```python
from build123d import *

# Parameters (mm, degrees)
SKETCH1_W                    = 44
SKETCH1_H                    = 210
BASE_FLANGE1_DEPTH           = 0.5
SKETCH6_R                    = 5
CUT_EXTRUDE1_DEPTH           = 108.281172626
LPATTERN1_COUNT              = 8
LPATTERN1_PITCH              = 25
EDGE_FLANGE1_STRIP_W         = 2.1
EDGE_FLANGE1_STRIP_H         = 0.5
EDGE_FLANGE1_STRIP_CUT_DEPTH = 210
EDGE_FLANGE1_DEPTH           = 210
F_7_0_7_DIAMETER_HOLE1_D     = 7
F_7_0_7_DIAMETER_HOLE1_DEPTH = 60
F_7_0_7_DIAMETER_HOLE1_TIP   = 2.103012167
BREAK_CORNER1_START          = 22
BREAK_CORNER1_DEPTH          = 0.5
CUT_EXTRUDE2_DEPTH           = 110.139818581
CUT_EXTRUDE2_DEPTH_BACK      = 110.139818581
SKETCH13_R                   = 3.1


# Read off the part's stored shape, not the designer's step: Break-Corner1
# Sheet-metal steps are written as plain solids
with BuildPart() as part:
    # Sketch1 → Base-Flange1 (new body)
    with BuildSketch(Plane.XY):
        Rectangle(SKETCH1_W, SKETCH1_H)
    extrude(amount=-BASE_FLANGE1_DEPTH)

    # Sketch6 → Cut-Extrude1 (cut, symmetric)
    with BuildSketch(Plane.XY):
        with Locations((10.825317547, 95)):
            Circle(SKETCH6_R)
        with Locations((-10.825317547, 82.5)):
            Circle(SKETCH6_R)
    cut_extrude1 = extrude(amount=CUT_EXTRUDE1_DEPTH, both=True, mode=Mode.SUBTRACT)

    # LPattern1: Cut-Extrude1 ×8
    with Locations(*[(0, -i * LPATTERN1_PITCH, 0) for i in range(1, LPATTERN1_COUNT)]):
        add(cut_extrude1, mode=Mode.SUBTRACT)

    # Edge-Flange1 strip (across the edge) → Edge-Flange1 strip cut (cut)
    with BuildSketch(Plane(origin=(22, -105, 0), x_dir=(-1, 0, 0), z_dir=(0, 1, 0))):
        with Locations((-1, -0.25)):
            Rectangle(EDGE_FLANGE1_STRIP_W, EDGE_FLANGE1_STRIP_H)
    extrude(amount=EDGE_FLANGE1_STRIP_CUT_DEPTH, mode=Mode.SUBTRACT)

    # Edge-Flange1 section (across the edge) → Edge-Flange1 (add)
    with BuildSketch(Plane(origin=(22, -105, 0), x_dir=(-1, 0, 0), z_dir=(0, 1, 0))):
        with BuildLine():
            Line((-0.5, 0.05), (-0.5, 19.5))
            Line((-0.5, 19.5), (0, 19.5))
            Line((0, 19.5), (0, 0.05))
            ThreePointArc((0, 0.05), (0.014644661, 0.014644661), (0.05, 0))
            Line((0.05, 0), (0.05, -0.5))
            ThreePointArc((0.05, -0.5), (-0.33890873, -0.33890873), (-0.5, 0.05))
        make_face()
    extrude(amount=EDGE_FLANGE1_DEPTH)

    # Ø7.0 (7) Diameter Hole1
    with Locations(Plane(origin=(22.5, 0, 0), x_dir=(0, 0, -1), z_dir=(1, 0, 0))):
        with Locations((-11.5, 95), (-11.5, -95)):
            Hole(F_7_0_7_DIAMETER_HOLE1_D / 2, depth=F_7_0_7_DIAMETER_HOLE1_DEPTH)
            with Locations((0, 0, -(F_7_0_7_DIAMETER_HOLE1_DEPTH + F_7_0_7_DIAMETER_HOLE1_TIP / 2))):  # 118° drill point
                Cone(0, F_7_0_7_DIAMETER_HOLE1_D / 2, F_7_0_7_DIAMETER_HOLE1_TIP, mode=Mode.SUBTRACT)

    # Break-Corner1 outline → Break-Corner1 (cut)
    with BuildSketch(Plane.YZ.offset(BREAK_CORNER1_START)):
        Polygon((-105, 19.5), (-105, 17.5), (-103, 19.5), align=None)
        Polygon((105, 19.5), (103, 19.5), (105, 17.5), align=None)
    extrude(amount=BREAK_CORNER1_DEPTH, mode=Mode.SUBTRACT)

    # Sketch13 → Cut-Extrude2 (cut, two sides: drawn at the far end of the back side and taken through both)
    with BuildSketch(Plane.XY.offset(-CUT_EXTRUDE2_DEPTH_BACK)):
        with Locations((-10.825317547, 95)):
            Circle(SKETCH13_R)
        with Locations((10.825317547, -92.5)):
            Circle(SKETCH13_R)
    extrude(amount=CUT_EXTRUDE2_DEPTH + CUT_EXTRUDE2_DEPTH_BACK, mode=Mode.SUBTRACT)


solid = part.part
```
CAD build for the part. Positions are in the model's coordinates, mm. Give positions to 0.01 mm unless a question says otherwise; leave off trailing zeros. Loops run counter-clockwise (first coordinate to the right, second up) from the corner with the lowest first, then second, coordinate; pieces in that order, holes last. Notation, with made-up numbers: (-31, 86.5) -> (3, 86.5) arc R15 cw to (3, 102.5) -> close; hole circle Ø5 at (21, 3). An arc over 180 degrees is marked (long way). Use a Markdown table: item, result.
1. Wall check: L1, parallel to X at y = -89.5, z = 15.5; L2, parallel to Z at x = 21, y = 79. Give the ranges that are in metal, low to high. Write a range as [from, to].
Check result:
| item | result |
|---|---|
| L1 | x = [22, 22.5] |
| L2 | z = [-0.5, 0] |
2. Slice it at B-B (z = 9.75). List the corners of the cut face in (x, y).
Check result:
| item | result |
|---|---|
| outline | (22, -105) -> (22.5, -105) -> (22.5, -98.03) -> (22, -98.03) -> close; (22, -91.97) -> (22.5, -91.97) -> (22.5, 91.97) -> (22, 91.97) -> close; (22, 98.03) -> (22.5, 98.03) -> (22.5, 105) -> (22, 105) -> close |
3. Mould opens along Z. For faces 1 (the cylindrical face through (-11.91, 27.62, -0.25)), 2 (the cylindrical face through (22.246, 91.583, 10.741)), 3 (the flat face through (0, 1, 0)), 4 (the flat face through (0, 1, -0.5)) say: pulls with the +Z half, pulls with the -Z half, needs draft (parallel to the pull), parting line crosses it, or undercut.
Check result:
| item | result |
|---|---|
| face 1 | needs draft |
| face 2 | undercut |
| face 3 | pulls with the +Z half |
| face 4 | pulls with the -Z half |
4. Slice it at C-C (x = 12). Give the number of separate pieces and of enclosed holes in the cut face, plus the area to 3 significant figures.
Check result:
| item | result |
|---|---|
| separate pieces | 10 |
| enclosed holes | 0 |
| area | 63.3 mm^2 |
5. Flat gauge pins, fed straight in: pin 1 (13 mm diameter, centred on x = -10.83, y = 7.5, fed in from +Z); pin 2 (16 mm diameter, centred on x = 10.83, y = 45, fed in from -Z); pin 3 (3 mm diameter, centred on y = 69.5, z = 3, fed in from -X). Where does each tip first touch, or does it go through?
Check result:
| item | result |
|---|---|
| pin 1 | stops at z = 0 |
| pin 2 | stops at z = -0.5 |
| pin 3 | stops at x = 22 |
6. Slice it at D-D (y = -7.5). List the corners of the cut face in (x, z).
Check result:
| item | result |
|---|---|
| outline | (-22, -0.5) -> (6.5, -0.5) -> (6.5, 0) -> (-22, 0) -> close; (15.16, -0.5) -> (21.95, -0.5) arc R0.55 ccw to (22.5, 0.05) -> (22.5, 19.5) -> (22, 19.5) -> (22, 0.05) arc R0.05 cw to (21.95, 0) -> (15.16, 0) -> close |
7. Slice it at A-A (y = 45). List the corners of the cut face in (x, z).
Check result:
| item | result |
|---|---|
| outline | (-22, -0.5) -> (5.83, -0.5) -> (5.83, 0) -> (-22, 0) -> close; (15.83, -0.5) -> (21.95, -0.5) arc R0.55 ccw to (22.5, 0.05) -> (22.5, 19.5) -> (22, 19.5) -> (22, 0.05) arc R0.05 cw to (21.95, 0) -> (15.83, 0) -> close |
